```python
from build123d import *

# Parameters (mm, degrees)
F1_DEPTH = 2.54
F2_R     = 5.08
F3_R     = 0.635
F4_DEPTH = 25.4
F5_W     = 22.621028
F5_H     = 7.478164
F6_DEPTH = 25.4
F7_R     = 5.08


with BuildPart() as f1:
    # F0 (on Front) → F1 (new body)
    with BuildSketch(Plane.XZ):
        Polygon((48.55294, 56.607572), (-65.74706, 56.607572), (-65.74706, 37.557572), (-53.04706, 37.557572), (-53.04706, 18.507572), (-65.74706, 18.507572), (-65.74706, -0.542428), (48.55294, -0.542428), (48.55294, 18.507572), (35.85294, 18.507572), (35.85294, 37.557572), (48.55294, 37.557572), align=None)
    extrude(amount=F1_DEPTH)

    # F2
    f2_edges = [f1.edges().sort_by_distance(p)[0] for p in [
        (-65.74706, -1.27, 56.607572),
        (-65.74706, -1.27, 37.557572),
        (-53.04706, -1.27, 37.557572),
        (-53.04706, -1.27, 18.507572),
        (-65.74706, -1.27, 18.507572),
        (-65.74706, -1.27, -0.542428),
        (48.55294, -1.27, -0.542428),
        (35.85294, -1.27, 18.507572),
        (48.55294, -1.27, 18.507572),
        (35.85294, -1.27, 37.557572),
        (48.55294, -1.27, 37.557572),
        (48.55294, -1.27, 56.607572),
    ]]
    fillet(f2_edges, radius=F2_R)

    # F3 (on face) → F4 (cut)
    with BuildSketch(Plane.XZ.offset(2.54)):
        with Locations((-42.918559, 1.362572)):
            Circle(F3_R)
        with Locations((-31.488559, 1.362572)):
            Circle(F3_R)
        with Locations((-20.058559, 1.362572)):
            Circle(F3_R)
        with Locations((-8.628559, 1.362572)):
            Circle(F3_R)
        with Locations((2.801441, 1.362572)):
            Circle(F3_R)
        with Locations((14.231441, 1.362572)):
            Circle(F3_R)
        with Locations((25.661441, 1.362572)):
            Circle(F3_R)
    extrude(amount=-F4_DEPTH, mode=Mode.SUBTRACT)

    # F5 (on face) → F6 (cut)
    with BuildSketch(Plane.XZ.offset(2.54)):
        with Locations((-11.923544, 52.86849)):
            Rectangle(F5_W, F5_H)
    extrude(amount=-F6_DEPTH, mode=Mode.SUBTRACT)

    # F7
    f7_edges = [f1.edges().sort_by_distance(p)[0] for p in [
        (-23.234058, -1.27, 49.129408),
        (-0.61303, -1.27, 49.129408),
    ]]
    fillet(f7_edges, radius=F7_R)


solid = f1.part
```
Work out the finished part from the listing and answer in its coordinate system (mm). A direction names the side the tool comes from. Round coordinates to 2 decimals unless told otherwise and drop trailing zeros. Write each loop counter-clockwise with the first axis right and the second up, starting at its lowest first coordinate (ties: lowest second). Pieces come first, ordered by that corner, then holes. Notation, with made-up numbers: (-30, 18.5) - (26, 18.5) arc R14 ccw to (26, 31.5) - close; hole circle Ø11 at (70, -10). An arc over 180 degrees is marked (long way). Return JSON: item names as keys, results as strings. Group by question number.
Q1. The part is cut by section B-B on y = -1.7. Count the separate pieces of the cut face and the enclosed holes in it, then the cut area to 3 significant figures.
Q2. The part is cut by section A-A on x = -13. Write down the section's boundary in (y, z), then the cut area to 3 significant figures.
Q3. For faces 5 (the cylindrical face through (-21.79, -1.25, 50.66)), 6 (the cylindrical face through (37.381, -1.288, 19.956)), 7 (the flat face through (-59, -1, 18.508)), determine the directions among +Z, -Z, +X, -X, +Y, -Y from which every point of the face is accessible in a straight line to the end or side of a thin tool.
Q4. The mould has two halves that part along X. Classify faces 1 (the cylindrical face through (-2.06, -1.25, 50.66)), 2 (the flat face through (-9, -1, -0.542)), 3 (the cylindrical face through (47.025, -1.288, 55.159)), 4 (the cylindrical face through (-64.22, -1.29, 55.16)): released by +X, released by -X, zero draft, split by the parting line, or undercut.
Q5. Each of these flat-tipped pins is pushed along its axis until it touches: pin 1 Ø1.1 at (x, z) = (25.66, 1.36) entering from -Y; pin 2 Ø1.2 at (y, z) = (-1.5, 55.5) entering from -X; pin 3 Ø0.8 at (y, z) = (-1, 27.5) entering from +X; pin 4 Ø0.7 at (y, z) = (-1.5, 56) entering from +X. Where does it stop, or does it pass through?
Q6. Find the intervals of material crossed by L1, parallel to X at y = -1.9, z = 23.5; L2, parallel to Z at x = -6, y = -0.3; L3, parallel to Z at x = -43, y = -1.4, in increasing order.
Solved:
{
 "1": {"separate pieces": "1", "enclosed holes": "7", "area": "5,860 mm²"},
 "2": {"outline": "(-2.54, -0.54) - (0, -0.54) - (0, 49.13) - (-2.54, 49.13) - close", "area": "126 mm²"},
 "3": {"face 5": "+Z, +Y, -Y", "face 6": "+X, +Y, -Y", "face 7": "-X, +Y, -Y"},
 "4": {"face 1": "undercut", "face 2": "zero draft", "face 3": "released by +X", "face 4": "released by -X"},
 "5": {"pin 1": "through", "pin 2": "x = -64.47", "pin 3": "x = 35.85", "pin 4": "x = 46.44"},
 "6": {"L1": "-53.05 to 35.85", "L2": "-0.54 to 49.13", "L3": "-0.54 to 0.73, 1.99 to 56.61"}
}
